```python
from build123d import *

# Parameters (mm, degrees)
F1_DEPTH = 8
F2_R     = 3.1
F3_DEPTH = 25


with BuildPart() as f1:
    # F0 (on Right) → F1 (new body)
    with BuildSketch(Plane.YZ):
        Polygon((0, -52), (0, 0), (7, 0), (7, 2), (-2, 2), (-2, -52), align=None)
    extrude(amount=F1_DEPTH)

    # F2 (on face) → F3 (cut)
    with BuildSketch(Plane.XZ.offset(2)):
        with Locations((4, -3.074622)):
            Circle(F2_R)
        with Locations((4, -38.02098)):
            Circle(F2_R)
    extrude(amount=-F3_DEPTH, mode=Mode.SUBTRACT)


solid = f1.part
```
Here's how the part is built. I have some questions about the finished solid (model axes, mm). A direction names the side the tool comes from. Coordinates: 2 decimals unless noted, no trailing zeros. Write each loop counter-clockwise with the first axis right and the second up, starting at its lowest first coordinate (ties: lowest second). Pieces come first, ordered by that corner, then holes. Notation, with made-up numbers: (-23, -10) - (31, -10) arc R25 ccw to (31, 11) - close; hole circle Ø11 at (20, 66.5). An arc over 180 degrees is marked (long way). One line per item, written item: value.
1) I'm going to push flat-ended pins straight in: P1, Ø1.5, axis at x = 5.5, z = -20.5, coming from the +Y side; P2, Ø1.1, axis at x = 2.5, y = 3.5, coming from the -Z side. Where does each tip first touch, or does it pass through?
Model answer:
P1: stops at y = 0
P2: stops at z = 0
2) Suppose I cut it at A-A on x = 1.5. Write out the boundary of the cut face in (y, z).
Model answer:
outline: (-2, -52) - (0, -52) - (0, -39.85) - (-2, -39.85) - close; (-2, -36.19) - (0, -36.19) - (0, -4.91) - (-2, -4.91) - close; (-2, -1.24) - (0, -1.24) - (0, 0) - (7, 0) - (7, 2) - (-2, 2) - close
3) I need wall thicknesses on line 1 along Z through (x, y) = (4, -1.2); line 2 along Z through (x, y) = (2.75, -0.5); line 3 along X through (y, z) = (-0.5, -3). Which ranges of each line are inside material? Lowest first, please.
Model answer:
line 1: z = -52 to -41.12, -34.92 to -6.17, 0.03 to 2
line 2: z = -52 to -40.86, -35.18 to -5.91, -0.24 to 2
line 3: x = 0 to 0.9, 7.1 to 8
4) Suppose I cut it at C-C on z = -13.5. Write out the boundary of the cut face in (x, y).
Model answer:
outline: (0, -2) - (8, -2) - (8, 0) - (0, 0) - close
5) We'd pull the mould along X, two halves only. Please class faces 1 (the cylindrical face through (4.226, -0.188, 0.017)), 2 (the flat face through (0, -1, -21)), 3 (the flat face through (2, 3, 0)): pulls with the +X half, pulls with the -X half, needs draft (parallel to the pull), parting line crosses it, or undercut.
Model answer:
face 1: undercut
face 2: pulls with the -X half
face 3: needs draft
6) Suppose I cut it at B-B on y = 1.75. Write out the boundary of the cut face in (x, z).
Model answer:
outline: (0, 0) - (3.6, 0) arc R3.1 cw to (4.4, 0) - (8, 0) - (8, 2) - (0, 2) - close
7) On a 3-axis mill with a long thin cutter (end or side, diameter ignored), from which of +Z, -Z, +X, -X, +Y, -Y can I reach the whole of each face in a straight line? I mean faces 4 (the flat face through (8, -1, -21)), 5 (the flat face through (4, 0, -26)). Say none if no direction works.
Model answer:
face 4: +Z, -Z, +X, +Y, -Y
face 5: -Z, +X, -X, +Y
